Geometry check sheet. Reference: the model listing, model coordinates, mm. Coordinates: 2 decimals unless noted, no trailing zeros. Write each loop counter-clockwise with the first axis right and the second up, starting at its lowest first coordinate (ties: lowest second). Pieces come first, ordered by that corner, then holes. Notation, with made-up numbers: M 13,73 L 63,73 A20 ccw 63,77 Z; hole C 22,-8.5 d2. An arc over 180 degrees is marked long. Write each question's results on one line, items separated by ' | '.
```python
from build123d import *

# Parameters (mm, degrees)
SKETCH2_R           = 6.35
BOSS_EXTRUDE1_DEPTH = 210


with BuildPart() as part:
    # Sketch2 → Boss-Extrude1 (new body)
    # profile 1 of 2: a face of its own
    with BuildSketch(Plane(origin=(0, 0, 0), x_dir=(1, 0, 0), z_dir=(0, 1, 0))):
        with BuildLine():
            Line((9.525, -34.717061728), (9.525, 0))
            Line((9.525, 0), (-9.525, 0))
            Line((-9.525, 0), (-9.525, -34.717061728))
            ThreePointArc((-9.525, -34.717061728), (0, -36), (9.525, -34.717061728))
        make_face()
        with Locations(Location((0, -17.358530864, 0), (0, 0, 270))):
            Circle(SKETCH2_R, mode=Mode.SUBTRACT)
    # profile 2 of 2: a face of its own
    with BuildSketch(Plane(origin=(0, 0, 0), x_dir=(1, 0, 0), z_dir=(0, 1, 0))):
        with BuildLine():
            Line((-9.525, 0), (9.525, 0))
            Line((9.525, 0), (9.525, 34.717061728))
            ThreePointArc((9.525, 34.717061728), (0, 36), (-9.525, 34.717061728))
            Line((-9.525, 34.717061728), (-9.525, 0))
        make_face()
        with Locations(Location((0, 17.358530864, 0), (0, 0, 270))):
            Circle(SKETCH2_R, mode=Mode.SUBTRACT)
    extrude(amount=BOSS_EXTRUDE1_DEPTH)


solid = part.part
```
Q1. Sectioned sample at C-C on y = 54. Record the cut outline in (x, z) (3 decimals).
Geometry check:
outline: M -9.525,-34.717 A36 ccw 9.525,-34.717 L 9.525,34.717 A36 ccw -9.525,34.717 Z; hole C 0,-17.359 d12.7; hole C 0,17.359 d12.7
Q2. Depth check by flat-ended pin: P1, Ø8, axis at x = 7, y = 76.5, coming from the +Z side; P2, Ø1, axis at x = -6.5, y = 76.5, coming from the -Z side. Enter the tip coordinate at first touch or a pass-through.
Geometry check:
P1: stops at z = 35.87 | P2: stops at z = -35.5
Q3. Sectioned sample at B-B on z = -13.5. Record the cut outline in (x, y) (3 decimals).
Geometry check:
outline: M -9.525,0 L -5.043,0 L -5.043,210 L -9.525,210 Z; M 5.043,0 L 9.525,0 L 9.525,210 L 5.043,210 Z
Q4. Mould release check, pull along X, two halves, no side actions. Record for faces 1 (the flat face through (9.525, 104, 0)), 2 (the flat face through (-9.525, 104, 0)), 3 (the cylindrical face through (1.9, 103.5, -11.3)), 4 (the cylindrical face through (1.907, 103.53, 23.415)): pulls with the +X half, pulls with the -X half, needs draft (parallel to the pull), parting line crosses it, or undercut.
Geometry check:
face 1: pulls with the +X half | face 2: pulls with the -X half | face 3: undercut | face 4: undercut
Q5. Sectioned sample at D-D on z = 16. Record the cut outline in (x, y) (3 decimals).
Geometry check:
outline: M -9.525,0 L -6.203,0 L -6.203,210 L -9.525,210 Z; M 6.203,0 L 9.525,0 L 9.525,210 L 6.203,210 Z
Q6. Sectioned sample at A-A on x = 0. Record the cut outline in (y, z), and give its area (3 significant figures).
Geometry check:
outline: M 0,-36 L 210,-36 L 210,-23.71 L 0,-23.71 Z; M 0,-11.01 L 210,-11.01 L 210,11.01 L 0,11.01 Z; M 0,23.71 L 210,23.71 L 210,36 L 0,36 Z | area: 9,790 mm2
Q7. Scan lines: probe 1 along Z at (x, y) = (1, 50.5); probe 2 along Z at (x, y) = (-4, 19.5); probe 3 along X at (y, z) = (52.5, -17.5) (3 decimals). Record each from-to range of solid material in increasing order.
Geometry check:
probe 1: z = -35.99 to -23.63, -11.09 to 11.09, 23.63 to 35.99 | probe 2: z = -35.78 to -22.29, -12.43 to 12.43, 22.29 to 35.78 | probe 3: x = -9.525 to -6.348, 6.348 to 9.525
